For this review, take the finished solid that the model builds, in its own axes (mm). A direction names the side the tool comes from. Coordinates: 2 decimals unless noted, no trailing zeros. Return JSON: item names as keys, results as strings. Group by question number.
Item 1: For line 1 along X through (y, z) = (46.5, 7.25); line 2 along Z through (x, y) = (-7.5, 83); line 3 along Z through (x, y) = (-34.5, 45), list the stretches that pass through material, from the lowest coordinate up.
Item 2: Take a section at A-A (z = 12). Count the separate pieces of the cut face and the enclosed holes in it, then the cut area to 3 significant figures.
Item 3: Insertion check: pin 1 (4 mm diameter, centred on x = -16, y = 72.5, fed in from -Z); pin 2 (0.7 mm diameter, centred on y = 46, z = 17.5, fed in from +X); pin 3 (1.4 mm diameter, centred on x = 4, y = 27.5, fed in from +Z); pin 4 (4 mm diameter, centred on y = 26, z = 14, fed in from -X). Each pin has a flat end and moves straight along its axis. Give the tip position at first contact, or say it passes through.
Item 4: Draft analysis for pull direction Z (two halves, no side actions). For faces 1 (the flat face through (3.11, 49.3, 15.2)), 2 (the flat face through (-3, 49, 18.9)), 3 (the flat face through (0.606, 49.3, 11.354)), 4 (the flat face through (-17.5, 49, 13)), state which applies: +Z half, -Z half, draft (parallel to the pull), parting line (faces both ways), or undercut.
Item 5: Machinability: for faces 5 (the flat face through (-23, 49, 9.1)), 6 (the flat face through (-33, 49, 9.7)), 7 (the flat face through (-12, 49, 18.9)), which of the approach directions +Z, -Z, +X, -X, +Y, -Y give a long, thin tool a straight path to every point of the face, cutting with its end or side? Answer none if there is none.
Autodesk Fusion 360 part; units mm, degrees
sketch "Skizze1" plane through (0, 0, 0) normal (0, 1, 0) x (1, 0, 0)
  line L0 (9.4, -17.7) -> (9.4, -18)
  line L1 (8.5, -17.7) -> (9.4, -17.7)
  line L2 (1.2293, -14.7) -> (0.1, -17.7)
  line L3 (4.3, -17.7) -> (4.3, -17.1)
  line L4 (0, -8.1) -> (1.2293, -14.7)
  line L5 (0.1, -18.9) -> (1.9, -18.9)
  line L6 (0.1, -17.7) -> (0.1, -18.9)
  line L7 (1.9, -18.4) -> (1.5, -18)
  line L8 (1.5, -18) -> (1.5, -17.7)
  line L9 (1.9, -18.9) -> (1.9, -18.4)
  line L10 (4.3, -17.1) -> (2.2465, -14.7)
  line L11 (13, 0) -> (0, 0)
  line L12 (9, -18.9) -> (11, -18.9)
  line L13 (0, 0) -> (0, -8.1)
  line L14 (8.5, -9.1) -> (8.5, -17.7)
  line L15 (4.3, -17.7) -> (1.5, -17.7)
  line L16 (11, -18.9) -> (11, -7.1)
  line L17 (9.4, -18) -> (9, -18.4)
  line L18 (9, -18.4) -> (9, -18.9)
  line L19 (4.9, -9.1) -> (2.0366, -9.1)
  line L20 (1.0172, -8.1) -> (2.2465, -14.7)
  line L21 (2.0366, -9.1) -> (1.0172, -8.1)
  line L22 (11, -7.1) -> (13, -7.1)
  line L23 (13, -7.1) -> (13, 0)
  circle A0 centre (12.5, -6.6) radius 0.5
  line L24 (2.2465, -14.7) -> (4, -15.7124)
  line L25 (2.2465, -14.7) -> (2.2465, -9.6844) construction
  line L26 (4.3, -17.1) -> (4, -15.7124)
  line L27 (0.7, -6.388) -> (0.7, -1)
  line L28 (0.7, -1) -> (12.5, -1)
  line L29 (12.5, -1) -> (12.5, -6.7)
  line L30 (12.5, -6.7) -> (10.6, -6.7)
  line L31 (10.6, -8.1) -> (10.6, -6.7)
  line L32 (4.9, -9.1) -> (4.9, -9.7)
  line L33 (4.9, -9.7) -> (7.9, -9.7)
  line L34 (7.9, -9.7) -> (7.9, -9.1)
  line L35 (7.9, -9.1) -> (8.5, -9.1)
  line L36 (8.5, -8.1) -> (10.6, -8.1)
  line L37 (1.7175, -7.3861) -> (0.7, -6.388)
  line L38 (6.9, -8.1) -> (8.5, -8.1)
  line L39 (6.9, -8.7) -> (6.9, -8.1)
  line L40 (5.9, -8.7) -> (6.9, -8.7)
  line L41 (5.9, -8.1) -> (5.9, -8.7)
  line L42 (5.9, -8.1) -> (2.4452, -8.1)
  line L43 (2.4452, -8.1) -> (1.7175, -7.3861)
  dimension "d14" = 7.9
  dimension "d15" = 2.8
  dimension "d16" = 0.9
  dimension "d17" = 17.7
  dimension "d18" = 0.3
  dimension "d21" = 18.9
  dimension "d26" = 35
  dimension "d28" = 1
  dimension "d30" = 150
  dimension "d31" = 0.4
  dimension "d32" = 1.4
  dimension "d33" = 1
  dimension "d34" = 0.6
  dimension "d35" = 3
  dimension "d36" = 45
  dimension "d37" = 45
  dimension "d38" = 0.4
  dimension "d39" = 0.1
  dimension "d42" = 1
  dimension "d94" = 2.5
  dimension "d95" = 0.5
  dimension "d96" = 0.5
  dimension "d97" = 2
  dimension "d98" = 1
  dimension "d105" = 120
  dimension "d106" = 2.5
  dimension "d119" = 8.6
  dimension "d135" = 1
  dimension "d136" = 0.7
  dimension "d137" = 0.5
  dimension "d139" = 0.4
  dimension "d141" = 0.4
  dimension "d142" = 0.6
  dimension "d143" = 0.6
  dimension "d144" = 8
  dimension "d146" = -1
extrude "Extrusion2" add sketch "Skizze1" along normal blind 1 contours A0 L29 L30 | A0 L29 L30
extrude "Extrusion1" add sketch "Skizze1" along normal blind 100
sketch "Skizze6" plane through (0, 0, 17.7) normal (0, 0, 1) x (-1, 0, 0)
  line L0 (-1.5, 0) -> (-4.3, 0)
  line L1 (-4.3, 0) -> (-4.3, -100)
  line L2 (-4.3, -100) -> (-1.5, -100)
  line L3 (-1.5, -100) -> (-1.5, 0)
  circle A0 centre (-3.25, -1.75) radius 0.75
  dimension "d99" = 1.5
  dimension "d100" = 1.75
  dimension "d102" = 1.75
sketch "Skizze4" plane through (0, 0, 0) normal (0, 0, -1) x (0, 1, 0)
  line L0 (0, 13) -> (0, 0)
  line L1 (100, 0) -> (100, 13)
  line L2 (0, 0) -> (0, 13)
  line L3 (0, 0) -> (-10, 0)
  line L4 (-10, 0) -> (-10, 13)
  line L5 (-10, 13) -> (0, 13)
  line L6 (50, 0) -> (50, 17.319) construction
  circle A0 centre (-5, 6.5) radius 1.65
  line L7 (100, 0) -> (110, 0)
  line L8 (100, 0) -> (100, 13)
  line L9 (110, 13) -> (100, 13)
  line L10 (110, 0) -> (110, 13)
  circle A1 centre (105, 6.5) radius 1.65
  line L11 (0, 0) -> (100, 0)
  line L12 (100, 13) -> (0, 13)
  circle A2 centre (105, 6.5) radius 4
  circle A3 centre (-5, 6.5) radius 4
  point P0 (-10, 6.5)
  point P1 (-5, 0)
  point P2 (0, 13)
  dimension "d88" = 3.3
  dimension "d89" = 10
  dimension "d123" = 8
pattern_linear "R-Anordnung1" count 4 spacing 13 along (-1, 0, 0) of "Extrusion1"
equation "Strip_width = 8 mm"
equation "Strip_hight = 0.3 mm"
equation "Reference_hight_machine = 18 mm"
equation "Length_Strips = 100 mm"
equation "Tape_Clearence = 0.1 mm"
equation "TapeSupport_width_HoleSide = 2.8 mm"
equation "TapeSupport_width_NonHoleSide = 0.9 mm"
equation "With_between_feeders = 2 mm"
equation "d14 = Strip_width - Tape_Clearence"
equation "d15 = TapeSupport_width_HoleSide"
equation "d16 = TapeSupport_width_NonHoleSide"
equation "d17 = Reference_hight_machine - Strip_hight"
equation "d18 = Strip_hight"
equation "d21 = Reference_hight_machine + 0.9 mm"
equation "d37 = d36"
equation "d38 = d31"
equation "d39 = Tape_Clearence"
equation "d40 = Length_Strips"
equation "d46 = -3 mm - Strip_width - With_between_feeders"
equation "width = 3 mm"
equation "d95 = d98 / 2"
equation "d96 = d98 / 2"
equation "d97 = With_between_feeders"
equation "Strip_Pitch = 4 mm"
equation "d102 = d100"
equation "d105 = 30 deg + 90 deg"
equation "Components_max_height = 8 mm"
equation "d141 = d139"
equation "d142 = d143"
equation "d144 = Components_max_height"
Findings below:
{
 "1": {"line 1": "x = -39 to -28, -26 to -15, -13 to -2, 0 to 11", "line 2": "z = 0 to 9.7", "line 3": "z = 0 to 9.1"},
 "2": {"separate pieces": "8", "enclosed holes": "0", "area": "1,410 mm2"},
 "3": {"pin 1": "stops at z = 0", "pin 2": "stops at x = 11", "pin 3": "stops at z = 17.7", "pin 4": "stops at x = -38.27"},
 "4": {"face 1": "undercut", "face 2": "+Z half", "face 3": "undercut", "face 4": "draft"},
 "5": {"face 5": "+Y, -Y", "face 6": "+Z, +Y, -Y", "face 7": "+Z, +X, -X, +Y, -Y"}
}
